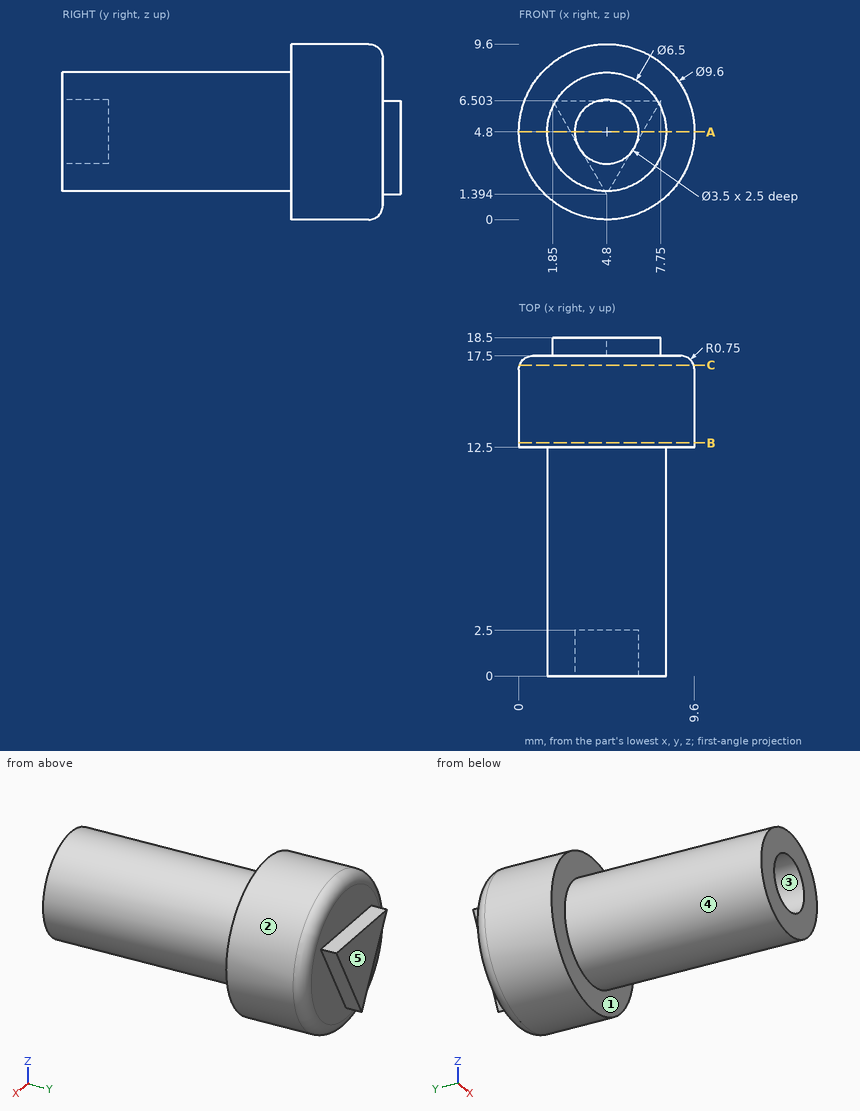
Design review of the part shown in the three views and the two pictorial views. Dimensions are in mm from the part's minimum x, y and z. A direction names the side the tool comes from. Give positions to 0.01 mm unless a question says otherwise; leave off trailing zeros. Loops run counter-clockwise (first coordinate to the right, second up) from the corner with the lowest first, then second, coordinate; pieces in that order, holes last. Notation, with made-up numbers: M -8.5,66.5 L 46.5,66.5 A24 cw 46.5,100.5 Z; hole C 12.25,35.25 d8. An arc over 180 degrees is marked long. Answer as a JSON object with one key per item and string values.
Item 1: We need section A-A (z = 4.8). State the section outline as (x, y) points.
Output values:
{"outline": "M 0,12.5 L 1.55,12.5 L 1.55,0 L 3.05,0 L 3.05,2.5 L 6.55,2.5 L 6.55,0 L 8.05,0 L 8.05,12.5 L 9.6,12.5 L 9.6,16.75 A0.75 ccw 8.85,17.5 L 6.77,17.5 L 6.77,18.5 L 2.83,18.5 L 2.83,17.5 L 0.75,17.5 A0.75 ccw 0,16.75 Z"}
Item 2: Machinability: for the marked faces 4 and 5, which of the approach directions +Z, -Z, +X, -X, +Y, -Y give a long, thin tool a straight path to every point of the face, cutting with its end or side? Answer none if there is none.
Output values:
{"face 4": "-Y", "face 5": "+Z, -Z, +X, -X, +Y"}
Item 3: Wall thickness on line 1 along Z through (x, y) = (4.8, 1.8); line 2 along Y through (x, z) = (5.75, 2.5); line 3 along Y through (x, z) = (3.5, 5.75): over which ranges is each line inside the solid? List them lowest first.
Output values:
{"line 1": "z = 1.55 to 3.05, 6.55 to 8.05", "line 2": "y = 0 to 17.5", "line 3": "y = 2.5 to 18.5"}
Item 4: Mouldability with a two-part tool opening along Z and no side actions: class the marked faces 1, 2 and 3 as pulls with the +Z half, pulls with the -Z half, needs draft (parallel to the pull), parting line crosses it, or undercut.
Output values:
{"face 1": "needs draft", "face 2": "parting line crosses it", "face 3": "undercut"}
Item 5: For P1, Ø3, axis at x = 4.8, z = 4.8, coming from the -Y side; P2, Ø1.5, axis at x = 4.5, y = 8, coming from the -Z side; P3, Ø1.5, axis at x = 3, y = 8, coming from the +Z side (1 decimal), all flat-tipped, find the tip position at first contact; note any pin that passes through.
Output values:
{"P1": "stops at y = 2.5", "P2": "stops at z = 1.55", "P3": "stops at z = 7.9"}
Item 6: We need section C-C (y = 17). State the section outline as (x, z) points, and give its area (3 significant figures).
Output values:
{"outline": "C 4.8,4.8 d9.51", "area": "71.1 mm2"}
Item 7: We need section B-B (y = 12.75). State the section outline as (x, z) points.
Output values:
{"outline": "C 4.8,4.8 d9.6"}
